Source: CAD feature listing. Evaluate the final solid. Frame: model axes, mm. Face numbers are marked on the shaded views. A direction names the side the tool comes from. Give positions to 0.01 mm unless a question says otherwise; leave off trailing zeros. Loops run counter-clockwise (first coordinate to the right, second up) from the corner with the lowest first, then second, coordinate; pieces in that order, holes last. Notation, with made-up numbers: (-9, 20.25) - (13, 20.25) arc R11 cw to (13, 26.25) - close; hole circle Ø5 at (-31, 30.5). An arc over 180 degrees is marked (long way). Write each question's results on one line, items separated by ' | '. Start each with the question number.
(1) Material intervals for line 1 along Y through (x, z) = (1.75, -2.5); line 2 along Y through (x, z) = (-5, -1.75); line 3 along Y through (x, z) = (-1, 2.5), sorted ascending. Write a range as [from, to].
(2) Cut plane C-C on x = 4.75. Return the cut outline in (y, z).
(3) Cut plane B-B on z = 3.75. Return the cut outline in (x, y), then the cut area to 3 significant figures.
(4) Reachability of the marked faces 1 and 2 from +Z, -Z, +X, -X, +Y, -Y: full face, straight path, thin tool, end or side. Return the list, or none.
(5) Cut plane A-A on y = 2.75. Return the cut outline in (x, z), then the cut area to 3 significant figures.
(6) Contact query for flat-ended pins moving along their axis: pin 1 (6 mm diameter, centred on x = 1.5, y = 4.5, fed in from +Z); pin 2 (6 mm diameter, centred on y = 2.5, z = -4.5, fed in from +X); pin 3 (6 mm diameter, centred on x = -1.5, y = -10, fed in from +Z); pin 4 (5 mm diameter, centred on x = 2, y = -7.5, fed in from +Z) (3 decimals). Output: stop coordinate, or through.
from build123d import *

# Parameters (mm, degrees)
SKETCH1_R           = 2.286
BOSS_EXTRUDE1_DEPTH = 7.88924
SKETCH2_R           = 2.38252
BOSS_EXTRUDE2_DEPTH = 4.762246
SKETCH3_R           = 3.175
BOSS_EXTRUDE3_DEPTH = 3.175
SKETCH4_R           = 3.175
BOSS_EXTRUDE4_DEPTH = 3.175
THREAD2_PITCH       = 1.27
SKETCH11_R          = 6.35
BOSS_EXTRUDE5_DEPTH = 3.81


with BuildPart() as part:
    # Sketch1 → Boss-Extrude1 (new body)
    with BuildSketch(Plane(origin=(0, 0, 0), x_dir=(1, 0, 0), z_dir=(0, 1, 0))):
        with Locations(Location((0, 0, 0), (0, 0, 270))):
            Circle(SKETCH1_R)
    extrude(amount=BOSS_EXTRUDE1_DEPTH)

    # Sketch2 → Boss-Extrude2 (add)
    with BuildSketch(Plane(origin=(0, 0, 0), x_dir=(-1, 0, 0), z_dir=(0, -1, 0))):
        with Locations(Location((0, 0, 0), (0, 0, 90))):
            Circle(SKETCH2_R)
    extrude(amount=BOSS_EXTRUDE2_DEPTH)

    # Sketch3 → Boss-Extrude3 (add)
    with BuildSketch(Plane(origin=(0, -4.762246, 0), x_dir=(-1, 0, 0), z_dir=(0, -1, 0))):
        with Locations(Location((0, 0, 0), (0, 0, 90))):
            Circle(SKETCH3_R)
    extrude(amount=BOSS_EXTRUDE3_DEPTH)

    # Sketch4 → Boss-Extrude4 (add)
    with BuildSketch(Plane(origin=(0, -7.937246, 0), x_dir=(-1, 0, 0), z_dir=(0, -1, 0))):
        with Locations(Location((0, 0, 0), (0, 0, 90))):
            Circle(SKETCH4_R)
    extrude(amount=BOSS_EXTRUDE4_DEPTH)

    # Thread2: the profile of Thread Profile3 profile screwed along a right-hand helix of 3.75 turns, 8 arcs to a turn; built about Z, then put on its axis
    thread2_z = Axis((0, 0, 0), (0, 0, 1))
    thread2_corners = [(3.1753, 0, -0.000173205), (3.1753, 0, 1.111423202), (2.487592339, 0, 0.714374998), (2.487592339, 0, 0.396874998)]
    with BuildLine(mode=Mode.PRIVATE) as thread2_profile:
        Line(thread2_corners[0], thread2_corners[1])
        Line(thread2_corners[1], thread2_corners[2])
        Line(thread2_corners[2], thread2_corners[3])
        Line(thread2_corners[3], thread2_corners[0])
    thread2_cap = Face(thread2_profile.wire())
    thread2_turn_angles = [0, 22.5, 45, 67.5, 90, 112.5, 135, 157.5, 180, 202.5, 225, 247.5, 270, 292.5, 315, 337.5, 360]
    thread2_turn_weights = [1, 0.9238795325112867, 1, 0.9238795325112867, 1, 0.9238795325112867, 1, 0.9238795325112867, 1, 0.9238795325112867, 1, 0.9238795325112867, 1, 0.9238795325112867, 1, 0.9238795325112867, 1]
    thread2_turn_rails = [Edge.make_bspline([Vector(p[0], p[1], 0).rotate(thread2_z, thread2_turn_angles[k]) / thread2_turn_weights[k] + Vector(0, 0, p[2] + THREAD2_PITCH * thread2_turn_angles[k] / 360) for k in range(17)], [0, 0, 0, 1, 1, 2, 2, 3, 3, 4, 4, 5, 5, 6, 6, 7, 7, 8, 8, 8], 2, thread2_turn_weights) for p in thread2_corners]
    thread2_turn_sides = [Face.make_surface_from_curves(thread2_turn_rails[p[0]], thread2_turn_rails[p[1]]) for p in [(0, 1), (1, 2), (2, 3), (3, 0)]]
    thread2_last_angles = [1080, 1102.5, 1125, 1147.5, 1170, 1192.5, 1215, 1237.5, 1260, 1282.5, 1305, 1327.5, 1350]
    thread2_last_weights = [1, 0.9238795325112867, 1, 0.9238795325112867, 1, 0.9238795325112867, 1, 0.9238795325112867, 1, 0.9238795325112867, 1, 0.9238795325112883, 1]
    thread2_last_rails = [Edge.make_bspline([Vector(p[0], p[1], 0).rotate(thread2_z, thread2_last_angles[k]) / thread2_last_weights[k] + Vector(0, 0, p[2] + THREAD2_PITCH * thread2_last_angles[k] / 360) for k in range(13)], [0, 0, 0, 1, 1, 2, 2, 3, 3, 4, 4, 5, 5, 6, 6, 6], 2, thread2_last_weights) for p in thread2_corners]
    thread2_last_sides = [Face.make_surface_from_curves(thread2_last_rails[p[0]], thread2_last_rails[p[1]]) for p in [(0, 1), (1, 2), (2, 3), (3, 0)]]
    thread2 = Plane(origin=(0, -9.524746, 0), x_dir=(1, 0, 0), z_dir=(0, 1, 0)) * Solid(Shell([*[p.moved(Location((0, 0, THREAD2_PITCH * i))) for i in range(3) for p in thread2_turn_sides], *thread2_last_sides, thread2_cap, thread2_cap.rotate(thread2_z, 1350).moved(Location((0, 0, THREAD2_PITCH * 1350 / 360)))]))
    add(thread2, mode=Mode.SUBTRACT)

    # Sketch11 → Boss-Extrude5 (add)
    with BuildSketch(Plane(origin=(0, -11.112246, 0), x_dir=(-1, 0, 0), z_dir=(0, -1, 0))):
        with Locations(Location((0, 0, 0), (0, 0, 270))):
            Circle(SKETCH11_R)
    extrude(amount=BOSS_EXTRUDE5_DEPTH)


solid = part.part
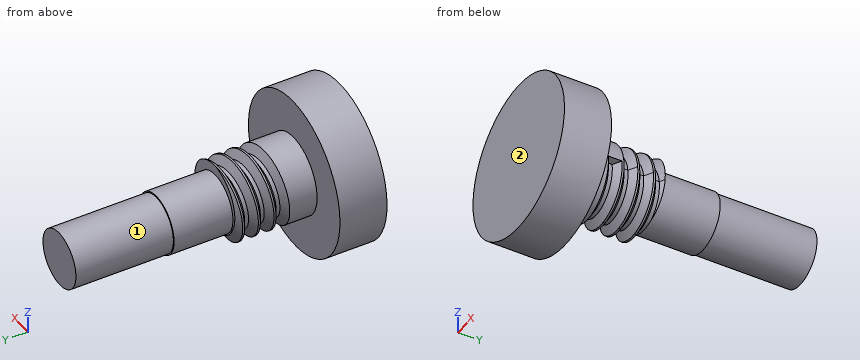
Ans:
1) line 1: [-14.92, -9.26], [-8.29, -7.99], [-7.02, -6.72], [-5.75, -5.45] | line 2: [-14.92, -11.11] | line 3: [-14.92, -8.37], [-7.82, -7.1], [-6.55, -5.83], [-5.28, -4.76]
2) outline: (-14.92, -4.21) - (-11.11, -4.21) - (-11.11, 4.21) - (-14.92, 4.21) - close
3) outline: (-5.12, -14.92) - (5.12, -14.92) - (5.12, -11.11) - (-5.12, -11.11) - close | area: 39.0 mm^2
4) face 1: +Y | face 2: +Z, -Z, +X, -X, -Y
5) outline: circle Ø4.57 at (0, 0) | area: 16.4 mm^2
6) pin 1: z = 2.29 | pin 2: x = 1.73 | pin 3: z = 6.35 | pin 4: z = 3.175
